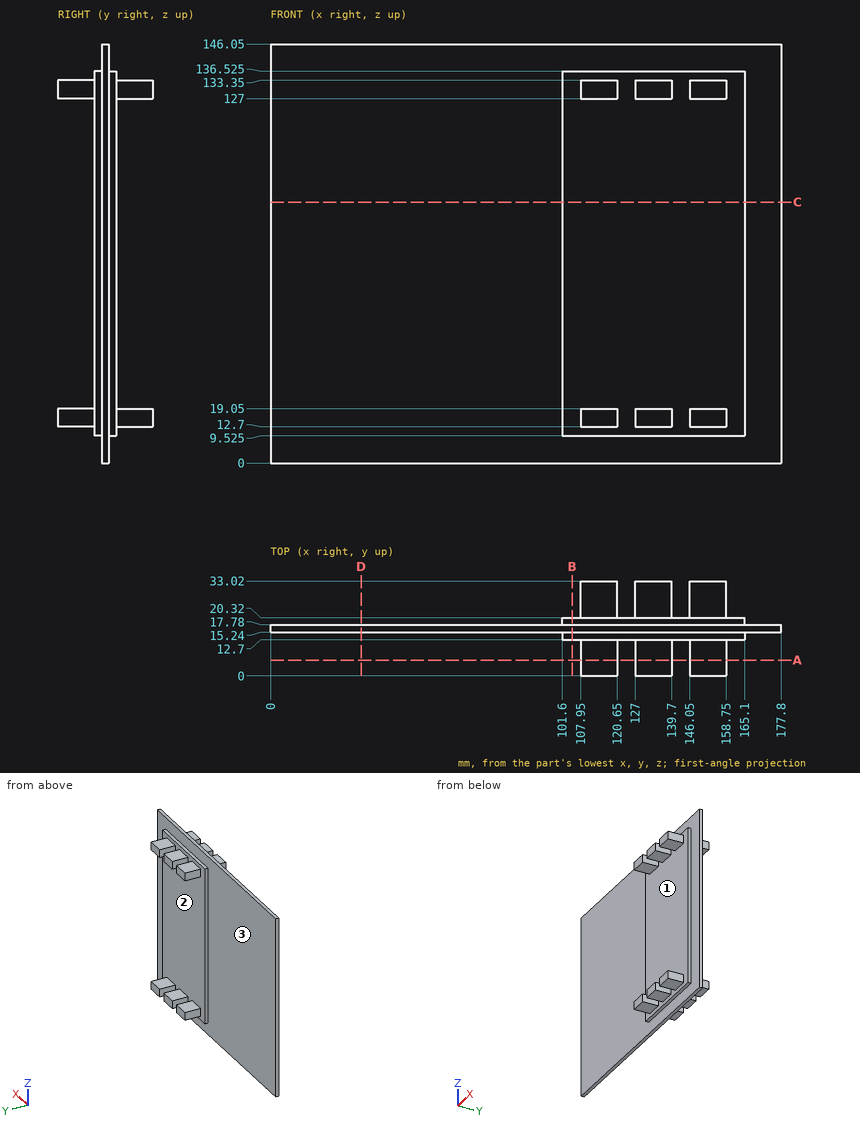
Job drawing, mm, ordinate dimensions from the low corner. One solid piece. Round coordinates to 2 decimals unless told otherwise and drop trailing zeros. Write each loop counter-clockwise with the first axis right and the second up, starting at its lowest first coordinate (ties: lowest second). Pieces come first, ordered by that corner, then holes. Notation, with made-up numbers: M -1.5,84.5 L 46.5,84.5 A25 ccw 46.5,109.5 Z; hole C -24,17.25 d4. An arc over 180 degrees is marked long. Return JSON: item names as keys, results as strings. Group by question number.
(1) Two-plate mould, pull along Z, no slides. Class the marked faces 1, 2 and 3: +Z half, -Z half, draft (parallel to the pull), parting line (faces both ways), or undercut.
(2) Saw through at A-A on y = 5.5. Write the cut outline in (x, z).
(3) Saw through at C-C on z = 91. Write the cut outline in (x, y).
(4) Pin check, flat tips, straight feed: pin 1 Ø14 at (x, y) = (152, 26) entering from +Z (3 decimals); pin 2 Ø3 at (y, z) = (25, 16) entering from +X; pin 3 Ø8 at (x, y) = (151, 26) entering from -Z; pin 4 Ø8 at (y, z) = (27.5, 118) entering from +X. Stop position of each tip, or through.
(5) Saw through at B-B on x = 105. Write the cut outline in (y, z) (3 decimals).
(6) Saw through at D-D on x = 31.5. Write the cut outline in (y, z), then the cut area to 3 significant figures.
(7) Drill centre lines: probe 1 along Z at (x, y) = (134, 7); probe 2 along X at (y, z) = (21, 128); probe 3 along X at (y, z) = (14, 57). Where is each one in solid material? Low to high.
Returned:
{
 "1": {"face 1": "undercut", "face 2": "undercut", "face 3": "draft"},
 "2": {"outline": "M 107.95,12.7 L 120.65,12.7 L 120.65,19.05 L 107.95,19.05 Z; M 107.95,127 L 120.65,127 L 120.65,133.35 L 107.95,133.35 Z; M 127,12.7 L 139.7,12.7 L 139.7,19.05 L 127,19.05 Z; M 127,127 L 139.7,127 L 139.7,133.35 L 127,133.35 Z; M 146.05,12.7 L 158.75,12.7 L 158.75,19.05 L 146.05,19.05 Z; M 146.05,127 L 158.75,127 L 158.75,133.35 L 146.05,133.35 Z"},
 "3": {"outline": "M 0,15.24 L 101.6,15.24 L 101.6,12.7 L 165.1,12.7 L 165.1,15.24 L 177.8,15.24 L 177.8,17.78 L 165.1,17.78 L 165.1,20.32 L 101.6,20.32 L 101.6,17.78 L 0,17.78 Z"},
 "4": {"pin 1": "z = 136.525", "pin 2": "x = 158.75", "pin 3": "z = 12.7", "pin 4": "through"},
 "5": {"outline": "M 12.7,9.525 L 15.24,9.525 L 15.24,0 L 17.78,0 L 17.78,9.525 L 20.32,9.525 L 20.32,136.525 L 17.78,136.525 L 17.78,146.05 L 15.24,146.05 L 15.24,136.525 L 12.7,136.525 Z"},
 "6": {"outline": "M 15.24,0 L 17.78,0 L 17.78,146.05 L 15.24,146.05 Z", "area": "371 mm²"},
 "7": {"probe 1": "12.7 to 19.05, 127 to 133.35", "probe 2": "107.95 to 120.65, 127 to 139.7, 146.05 to 158.75", "probe 3": "101.6 to 165.1"}
}
